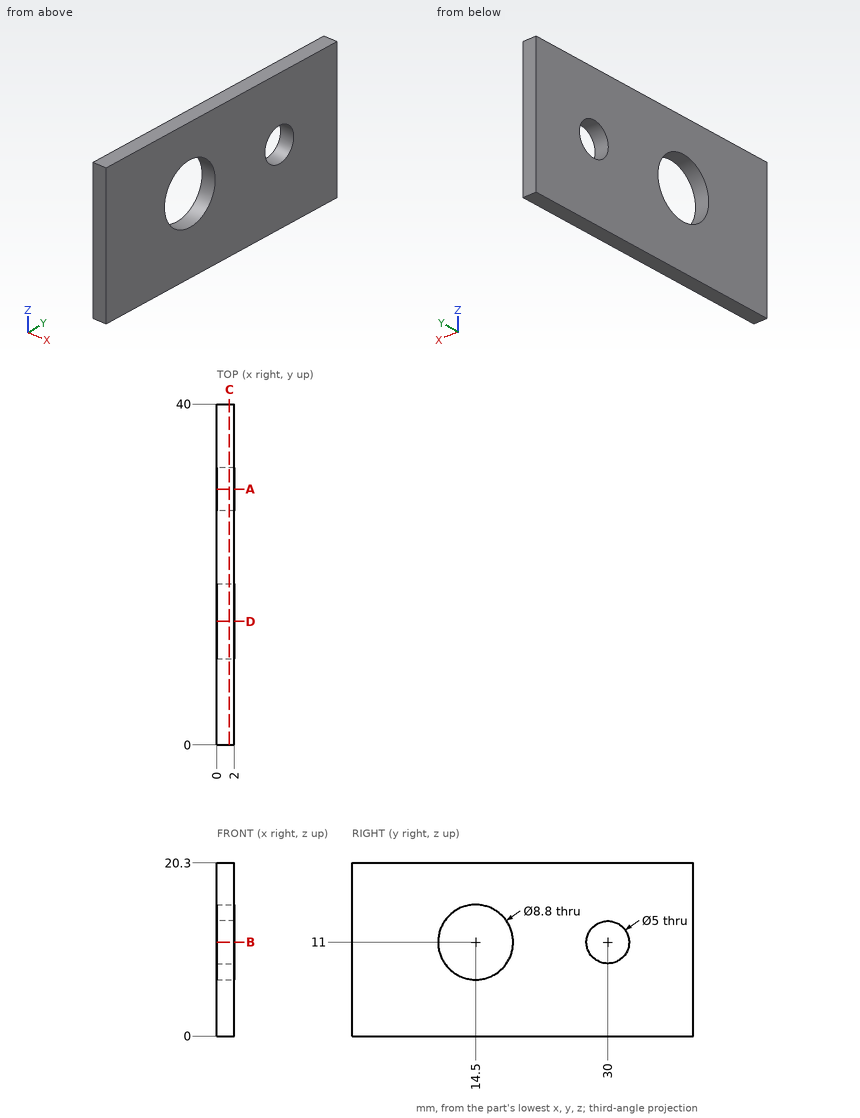
Job drawing, mm, ordinate dimensions from the low corner. One solid piece. Round coordinates to 2 decimals unless told otherwise and drop trailing zeros. Loops run counter-clockwise (first coordinate to the right, second up) from the corner with the lowest first, then second, coordinate; pieces in that order, holes last.
(1) Cut at D-D (y = 14.5). Give the cut face in (x, z).
(2) Cut at C-C (x = 1.45). Give the cut face in (y, z).
(3) Drop a flat-ended pin along its axis: pin 1 (1.5 mm diameter, centred on y = 29.5, z = 12, fed in from -X). Give the stop position or say it passes through.
(4) Cut at A-A (y = 30). Give the cut face in (x, z), plus the area to 3 significant figures.
(5) Cut at B-B (z = 11). Give the cut face in (x, y).
(6) Wall check: line 1 along Y through (x, z) = (0.7, 11); line 2 along Z through (x, y) = (1.4, 30); line 3 along Z through (x, y) = (0.45, 13.5). Give the ranges that are in metal, low to high.
Findings below:
1. outline: (0, 0) - (2, 0) - (2, 6.6) - (0, 6.6) - close; (0, 15.4) - (2, 15.4) - (2, 20.3) - (0, 20.3) - close
2. outline: (0, 0) - (40, 0) - (40, 20.3) - (0, 20.3) - close; hole circle Ø8.8 at (14.5, 11); hole circle Ø5 at (30, 11)
3. pin 1: passes through
4. outline: (0, 0) - (2, 0) - (2, 8.5) - (0, 8.5) - close; (0, 13.5) - (2, 13.5) - (2, 20.3) - (0, 20.3) - close
4. area: 30.6 mm2
5. outline: (0, 0) - (2, 0) - (2, 10.1) - (0, 10.1) - close; (0, 18.9) - (2, 18.9) - (2, 27.5) - (0, 27.5) - close; (0, 32.5) - (2, 32.5) - (2, 40) - (0, 40) - close
6. line 1: y = 0 to 10.1, 18.9 to 27.5, 32.5 to 40
6. line 2: z = 0 to 8.5, 13.5 to 20.3
6. line 3: z = 0 to 6.72, 15.28 to 20.3
